Geometry: final body of the model. Coordinates: model frame, mm. A direction names the side the tool comes from. Coordinates: 2 decimals unless noted, no trailing zeros. Order: outer loops, then holes, each group sorted by start corner. A loop starts at its lowest first (then second) coordinate and runs counter-clockwise, first axis right, second up. Notation, with made-up numbers: M -34,88.5 L -3,88.5 A20 ccw -3,106.5 Z; hole C 70.25,-26 d10. An arc over 180 degrees is marked long. One line per question, with ' | ' between items.
from build123d import *

# Parameters (mm, degrees)
PAD_DEPTH    = 1
SKETCH002_W  = 0.4
SKETCH002_H  = 0.4
PAD001_DEPTH = 6
SKETCH003_W  = 2.84
SKETCH003_H  = 0.4
PAD002_DEPTH = 1


with BuildPart() as pad:
    # Sketch001 → Pad (new body)
    with BuildSketch(Plane(origin=(1.27, 0, 3), x_dir=(1, 0, 0), z_dir=(0, 0, 1))):
        with BuildLine():
            ThreePointArc((-1.5, -1.16619), (1.9, 0), (-1.5, 1.16619))
            Line((-1.5, -1.16619), (-1.5, 1.16619))
        make_face()
    extrude(amount=PAD_DEPTH)


with BuildPart() as pad001:
    # Sketch002 → Pad001 (new body)
    with BuildSketch(Plane.XY.offset(3.5)):
        Rectangle(SKETCH002_W, SKETCH002_H)
        with Locations((2.54, 0)):
            Rectangle(SKETCH002_W, SKETCH002_H)
    extrude(amount=-PAD001_DEPTH)


with BuildPart() as pad002:
    # Sketch003 → Pad002 (new body)
    with BuildSketch(Plane.XY.offset(3.5)):
        with Locations((1.27, 0)):
            Rectangle(SKETCH003_W, SKETCH003_H)
    extrude(amount=PAD002_DEPTH)


with BuildPart() as revolution001:
    # Sketch004 → Revolution001 (revolve)
    with BuildSketch(Plane.XZ):
        Polygon((1.27, 4.275), (0.82, 4.725), (1.27, 4.725), align=None)
    revolve(axis=Axis((1.27, 0, 5.374987), (0, 0, -1)))


with BuildPart() as led_d3_0mm:
    # Sketch → Revolution (revolve)
    with BuildSketch(Plane(origin=(1.27, 0, 0), x_dir=(1, 0, 0), z_dir=(0, -1, 0))):
        with BuildLine():
            ThreePointArc((1.45, 6.85), (1.025305, 7.875305), (0, 8.3))
            Line((0, 4), (0, 8.3))
            Line((1.45, 4), (0, 4))
            Line((1.45, 6.85), (1.45, 4))
        make_face()
    revolve(axis=Axis((1.27, 0, 0), (0, 0, 1)))

    add(pad.part)
    add(pad001.part)
    add(pad002.part)
    add(revolution001.part)


solid = led_d3_0mm.part
1. Pin query (flat end, axial travel): P1, Ø1, axis at x = 1, y = 0, coming from the -Z side; P2, Ø1.5, axis at y = 0, z = 2, coming from the +X side. Return the tip coordinate at first contact, or that it passes through.
Response values:
P1: stops at z = 3 | P2: stops at x = 2.74
2. Access query for faces 1 (the face through (-0.23, 0, 3.5)), 2 (the face through (2.65, 0.44, 5.41)). Directions: +Z, -Z, +X, -X, +Y, -Y. A direction counts if a zero-diameter tool reaches every point of the face in a straight line with its end or side. Return the directions, or none.
Response values:
face 1: +Z, -Z, -X, +Y, -Y | face 2: +Z
3. Material intervals for line 1 (Z direction, x = 2.9, y = -0.25); line 2 (Y direction, x = 2.55, z = 1.25); line 3 (Y direction, x = 0.6, z = 4.25), sorted ascending. Write a range as [from, to].
Response values:
line 1: z = [3, 4] | line 2: y = [-0.2, 0.2] | line 3: y = [-1.29, 1.29]
4. Section B-B, the plane z = 5.75. Output: boundary loops of the cut face in (x, y).
Response values:
outline: C 1.27,0 d2.9
5. Section A-A, the plane z = -1.5. Output: boundary loops of the cut face in (x, y), and give its area (3 significant figures).
Response values:
outline: M -0.2,-0.2 L 0.2,-0.2 L 0.2,0.2 L -0.2,0.2 Z; M 2.34,-0.2 L 2.74,-0.2 L 2.74,0.2 L 2.34,0.2 Z | area: 0.320 mm^2
